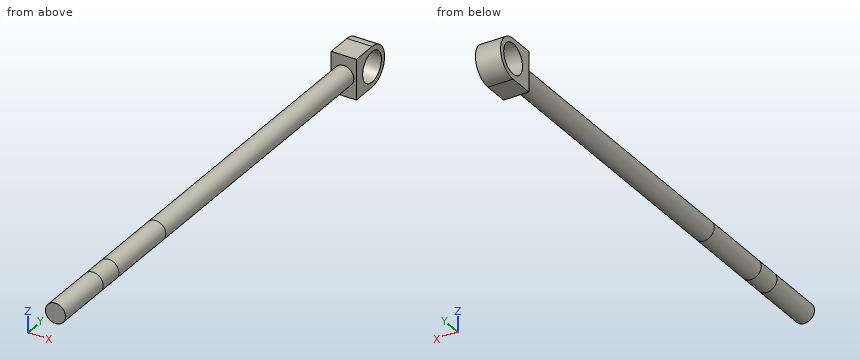
```python
from build123d import *

# Parameters (mm, degrees)
SKETCH_1_R       = 2
EXTRUDE_1_DEPTH  = 60
SKETCH_8_R       = 3
EXTRUDE_8_DEPTH  = 2.5
EXTRUDE_START    = 15
SKETCH_9_R       = 2
EXTRUDE_9_DEPTH  = 15
EXTRUDE_START_2  = 5
SKETCH_12_R      = 2
EXTRUDE_11_DEPTH = 5
EXTRUDE_START_3  = 17
SKETCH_10_R      = 2
EXTRUDE_10_DEPTH = 12


with BuildPart() as part:
    # Sketch 1 → Extrude 1 (new body)
    with BuildSketch(Plane(origin=(0, 0, 0), x_dir=(1, 0, 0), z_dir=(0, 1, 0))):
        with Locations(Location((0, 0, 0), (0, 0, 270))):
            Circle(SKETCH_1_R)
    extrude(amount=EXTRUDE_1_DEPTH)

    # Sketch 8 → Extrude 8 (add, symmetric)
    with BuildSketch(Plane(origin=(0, 0, 0), x_dir=(0, 0, -1), z_dir=(1, 0, 0))):
        with BuildLine():
            Line((-4, 65), (-4, 60))
            Line((-4, 60), (4, 60))
            Line((4, 60), (4, 65))
            ThreePointArc((4, 65), (0, 69), (-4, 65))
        make_face()
        with Locations((0, 65)):
            Circle(SKETCH_8_R, mode=Mode.SUBTRACT)
    extrude(amount=EXTRUDE_8_DEPTH, both=True)

    # Sketch 9 → Extrude 9 (add)
    with BuildSketch(Plane.XZ.offset(EXTRUDE_START)):
        with Locations(Location((0, 0, 0), (0, 0, 270))):
            Circle(SKETCH_9_R)
    extrude(amount=-EXTRUDE_9_DEPTH)

    # Sketch 12 → Extrude 11 (add)
    with BuildSketch(Plane.XZ.offset(15).offset(EXTRUDE_START_2)):
        with Locations(Location((0, 0, 0), (0, 0, 270))):
            Circle(SKETCH_12_R)
    extrude(amount=-EXTRUDE_11_DEPTH)

    # Sketch 10 → Extrude 10 (add)
    with BuildSketch(Plane.XZ.offset(15).offset(EXTRUDE_START_3)):
        with Locations(Location((0, 0, 0), (0, 0, 270))):
            Circle(SKETCH_10_R)
    extrude(amount=-EXTRUDE_10_DEPTH)


solid = part.part
```
Part model, mm, in its own coordinate system. Round coordinates to 2 decimals unless told otherwise and drop trailing zeros. Write each loop counter-clockwise with the first axis right and the second up, starting at its lowest first coordinate (ties: lowest second). Pieces come first, ordered by that corner, then holes. Notation, with made-up numbers: (32, 18) -> (81, 18) arc R24 cw to (81, 29) -> close; hole circle Ø2 at (5, 13). An arc over 180 degrees is marked (long way). Return JSON: item names as keys, results as strings. Group by question number.
Q1. Saw through at C-C on y = -24. Write the cut outline in (x, z).
Q2. Saw through at B-B on x = 0. Write the cut outline in (y, z), plus the area to 3 significant figures.
Q3. Pin check, flat tips, straight feed: pin 1 (4 mm diameter, centred on y = -7.5, z = -0.5, fed in from +X); pin 2 (1.5 mm diameter, centred on y = -3, z = -1, fed in from -X); pin 3 (2 mm diameter, centred on x = 1, y = 24, fed in from -Z). Stop position of each tip, or through.
Q4. Probe L1, parallel to Y at x = 0.6, z = 0.25; L2, parallel to Y at x = -0.8, z = 1.25; L3, parallel to Z at x = -0.2, y = -6. List the from-to ranges inside material, lowest first. Write a range as [from, to].
Q5. Saw through at A-A on z = 0. Write the cut outline in (x, y).
Answer:
{
 "1": {"outline": "circle Ø4 at (0, 0)"},
 "2": {"outline": "(-32, -2) -> (60, -2) -> (60, -4) -> (65, -4) arc R4 ccw to (65, 4) -> (60, 4) -> (60, 2) -> (-32, 2) -> close; hole circle Ø6 at (65, 0)", "area": "405 mm2"},
 "3": {"pin 1": "x = 2", "pin 2": "x = -1.98", "pin 3": "z = -2"},
 "4": {"L1": "[-32, 62.01], [67.99, 68.99]", "L2": "[-32, 62.27], [67.73, 68.8]", "L3": "[-1.99, 1.99]"},
 "5": {"outline": "(-2.5, 60) -> (-2, 60) -> (-2, -32) -> (2, -32) -> (2, 60) -> (2.5, 60) -> (2.5, 62) -> (-2.5, 62) -> close; (-2.5, 68) -> (2.5, 68) -> (2.5, 69) -> (-2.5, 69) -> close"}
}
